Design review of the part built by this model. Coordinates are the model's own, in mm. Coordinates: 2 decimals unless noted, no trailing zeros. Order: outer loops, then holes, each group sorted by start corner. A loop starts at its lowest first (then second) coordinate and runs counter-clockwise, first axis right, second up. Notation, with made-up numbers: M 33.5,10 L 88.5,10 A30 ccw 88.5,38 Z; hole C -15,37.5 d1. An arc over 180 degrees is marked long. Use CSV: the item, a comma, the result in double quotes.
```python
from build123d import *

# Parameters (mm, degrees)
SKETCH1_W                            = 254
SKETCH1_H                            = 228.6
BASE_PLATE_DEPTH                     = 6.35
SLOTS_DEPTH                          = 7.35
FEET_CONNECTION_HOLE_D               = 8.7376
HOLE_FOR_10_BLIND_FASTENERS_B_BS_1_D = 6.35


with BuildPart() as part:
    # Sketch1 → base plate (new body)
    with BuildSketch(Plane(origin=(0, 0, 0), x_dir=(1, 0, 0), z_dir=(0, 1, 0))):
        with Locations((127, -114.3)):
            Rectangle(SKETCH1_W, SKETCH1_H)
    extrude(amount=-BASE_PLATE_DEPTH)

    # Sketch3 → slots (cut, through all)
    with BuildSketch(Plane(origin=(0, 0, 0), x_dir=(1, 0, 0), z_dir=(0, 1, 0))):
        with BuildLine():
            ThreePointArc((59.421325374, -43.892898159), (59.421325374, -46.721325374), (56.592898159, -46.721325374))
            Line((56.592898159, -46.721325374), (51.204744487, -41.333171702))
            ThreePointArc((51.204744487, -41.333171702), (51.204744487, -38.504744487), (54.033171702, -38.504744487))
            Line((54.033171702, -38.504744487), (59.421325374, -43.892898159))
        make_face()
        with BuildLine():
            Line((199.966828298, -38.504744487), (194.578674626, -43.892898159))
            ThreePointArc((194.578674626, -43.892898159), (194.578674626, -46.721325374), (197.407101841, -46.721325374))
            Line((197.407101841, -46.721325374), (202.795255513, -41.333171702))
            ThreePointArc((202.795255513, -41.333171702), (202.795255513, -38.504744487), (199.966828298, -38.504744487))
        make_face()
        with BuildLine():
            Line((185.598418504, -58.530008711), (190.986572177, -53.141855038))
            ThreePointArc((190.986572177, -53.141855038), (190.986572177, -50.313427823), (188.158144962, -50.313427823))
            Line((188.158144962, -50.313427823), (182.769991289, -55.701581496))
            ThreePointArc((182.769991289, -55.701581496), (182.769991289, -58.530008711), (185.598418504, -58.530008711))
        make_face()
        with BuildLine():
            ThreePointArc((190.986572177, -175.458144962), (190.986572177, -178.286572177), (188.158144962, -178.286572177))
            Line((188.158144962, -178.286572177), (182.769991289, -172.898418504))
            ThreePointArc((182.769991289, -172.898418504), (182.769991289, -170.069991289), (185.598418504, -170.069991289))
            Line((185.598418504, -170.069991289), (190.986572177, -175.458144962))
        make_face()
        with BuildLine():
            ThreePointArc((194.578674626, -184.707101841), (194.578674626, -181.878674626), (197.407101841, -181.878674626))
            Line((197.407101841, -181.878674626), (202.795255513, -187.266828298))
            ThreePointArc((202.795255513, -187.266828298), (202.795255513, -190.095255513), (199.966828298, -190.095255513))
            Line((199.966828298, -190.095255513), (194.578674626, -184.707101841))
        make_face()
        with BuildLine():
            Line((54.033171702, -190.095255513), (59.421325374, -184.707101841))
            ThreePointArc((59.421325374, -184.707101841), (59.421325374, -181.878674626), (56.592898159, -181.878674626))
            Line((56.592898159, -181.878674626), (51.204744487, -187.266828298))
            ThreePointArc((51.204744487, -187.266828298), (51.204744487, -190.095255513), (54.033171702, -190.095255513))
        make_face()
        with BuildLine():
            Line((68.401581496, -170.069991289), (63.013427823, -175.458144962))
            ThreePointArc((63.013427823, -175.458144962), (63.013427823, -178.286572177), (65.841855038, -178.286572177))
            Line((65.841855038, -178.286572177), (71.230008711, -172.898418504))
            ThreePointArc((71.230008711, -172.898418504), (71.230008711, -170.069991289), (68.401581496, -170.069991289))
        make_face()
        with BuildLine():
            Line((68.401581496, -58.530008711), (63.013427823, -53.141855038))
            ThreePointArc((63.013427823, -53.141855038), (63.013427823, -50.313427823), (65.841855038, -50.313427823))
            Line((65.841855038, -50.313427823), (71.230008711, -55.701581496))
            ThreePointArc((71.230008711, -55.701581496), (71.230008711, -58.530008711), (68.401581496, -58.530008711))
        make_face()
    extrude(amount=-SLOTS_DEPTH, mode=Mode.SUBTRACT)

    # Feet connection hole (through all)
    with Locations(Plane(origin=(0, 0, 0), x_dir=(1, 0, 0), z_dir=(0, 1, 0))):
        with Locations((12.7, -215.9), (241.3, -12.7), (12.7, -12.7), (241.3, -215.9)):
            Hole(FEET_CONNECTION_HOLE_D / 2)

    # Hole for #10 Blind Fasteners (B,BS)1 (through all)
    with Locations(Plane(origin=(0, 0, 0), x_dir=(1, 0, 0), z_dir=(0, 1, 0))):
        with Locations((127, -215.9), (127, -12.7)):
            Hole(HOLE_FOR_10_BLIND_FASTENERS_B_BS_1_D / 2)


solid = part.part
```
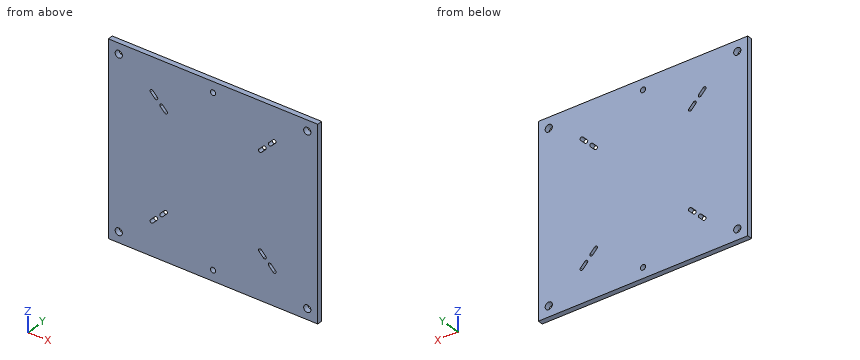
(1) Add section A-A on z = 215.9. State the section outline as (x, y) points (3 decimals).
The answers:
outline,"M 0,-6.35 L 8.331,-6.35 L 8.331,0 L 0,0 Z; M 17.069,-6.35 L 123.825,-6.35 L 123.825,0 L 17.069,0 Z; M 130.175,-6.35 L 236.931,-6.35 L 236.931,0 L 130.175,0 Z; M 245.669,-6.35 L 254,-6.35 L 254,0 L 245.669,0 Z"
(2) Wall thickness on probe 1 along X at (y, z) = (-2, 215.9) (3 decimals); probe 2 along Z at (x, y) = (12.7, -1.75); probe 3 along Z at (x, y) = (127, -2.75) (3 decimals): over which ranges is each line inside the solid? List them lowest first.
The answers:
probe 1,"x = 0 to 8.331, 17.069 to 123.825, 130.175 to 236.931, 245.669 to 254"
probe 2,"z = 0 to 8.33, 17.07 to 211.53, 220.27 to 228.6"
probe 3,"z = 0 to 9.525, 15.875 to 212.725, 219.075 to 228.6"
(3) Add section B-B on x = 127. State the section outline as (y, z) points (3 decimals).
The answers:
outline,"M -6.35,0 L 0,0 L 0,9.525 L -6.35,9.525 Z; M -6.35,15.875 L 0,15.875 L 0,212.725 L -6.35,212.725 Z; M -6.35,219.075 L 0,219.075 L 0,228.6 L -6.35,228.6 Z"
(4) Add section C-C on x = 241.3. State the section outline as (y, z) points, and give its area (3 significant figures).
The answers:
outline,"M -6.35,0 L 0,0 L 0,8.33 L -6.35,8.33 Z; M -6.35,17.07 L 0,17.07 L 0,211.53 L -6.35,211.53 Z; M -6.35,220.27 L 0,220.27 L 0,228.6 L -6.35,228.6 Z"
area,"1,340 mm2"
